Answer from the drawing. Dimensions are ordinates in mm from the lowest x, y and z of the part. A direction names the side the tool comes from. Give positions to 0.01 mm unless a question says otherwise; leave off trailing zeros. Write each loop counter-clockwise with the first axis right and the second up, starting at its lowest first coordinate (ties: lowest second). Pieces come first, ordered by that corner, then holes. Notation, with made-up numbers: M 75.5,9.25 L 131.5,9.25 A12 ccw 131.5,20.25 Z; hole C -14.5,5 d10. An arc over 180 degrees is marked long. Put each result on its own line as item: value.
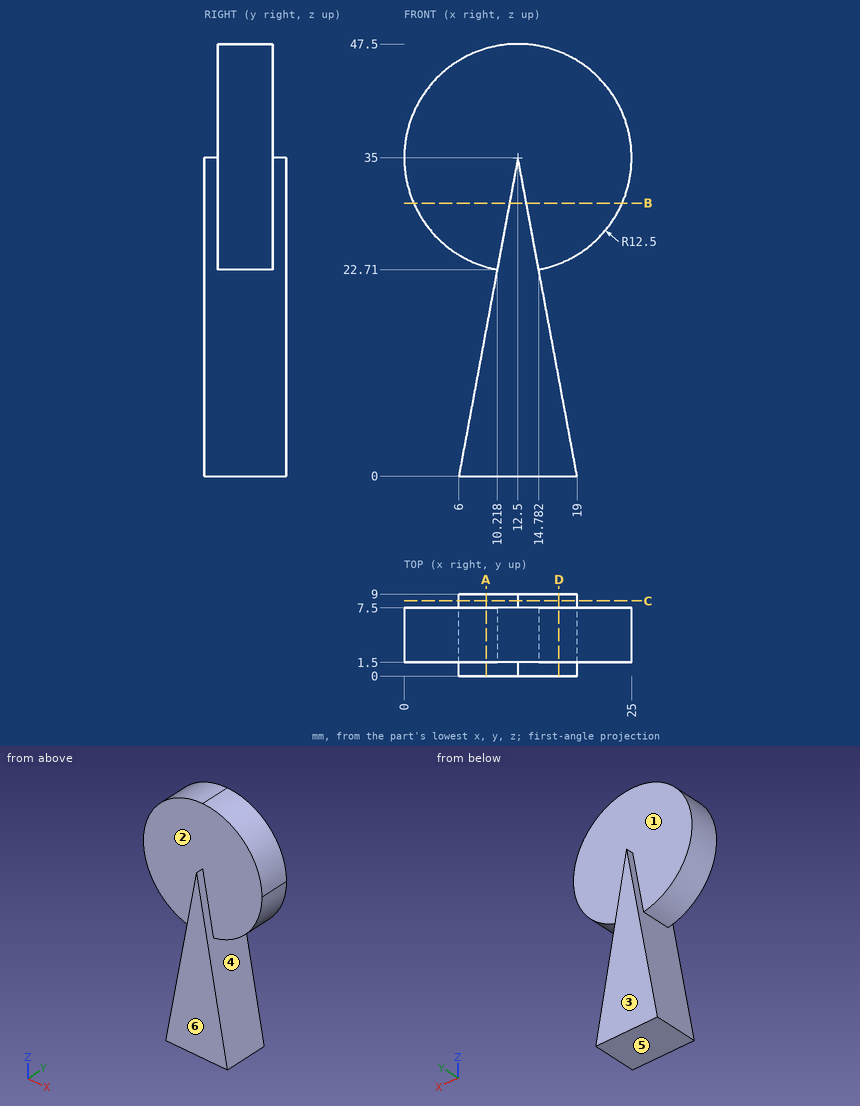
(1) Section C-C on y = 8.25 is taken. Determine the outline of the cut face in (x, z).
Result:
outline: M 6,0 L 19,0 L 12.5,35 Z
(2) Straight lines are drawn through the part: line 1 along Y through (x, z) = (6, 25.5); line 2 along Z through (x, y) = (12, 6.5); line 3 along Z through (x, y) = (22.5, 3.25). For each, find the intervals that lie inside material, in ascending order. Write a range as from..to.
Result:
line 1: y = 1.5..7.5
line 2: z = 0..47.49
line 3: z = 27.5..42.5
(3) Section B-B on z = 30 is taken. Determine the outline of the cut face in (x, y), and give its area (3 significant figures).
Result:
outline: M 1.04,1.5 L 11.57,1.5 L 11.57,0 L 13.43,0 L 13.43,1.5 L 23.96,1.5 L 23.96,7.5 L 13.43,7.5 L 13.43,9 L 11.57,9 L 11.57,7.5 L 1.04,7.5 Z
area: 143 mm²
(4) Which of the six approach directions +Z, -Z, +X, -X, +Y, -Y give full straight-line access (tool end or side, diameter ignored) to the marked faces 1, 2 and 3?
Result:
face 1: +Z, +Y
face 2: +Z, -Y
face 3: +Z, -Z, +X, -X, +Y
(5) Section D-D on x = 17 is taken. Determine the outline of the cut face in (y, z).
Result:
outline: M 0,0 L 9,0 L 9,10.77 L 0,10.77 Z; M 1.5,23.34 L 7.5,23.34 L 7.5,46.66 L 1.5,46.66 Z
(6) For a pull along Z with two mould halves and no side action, classify the marked faces 4, 5 and 6 as +Z half, -Z half, draft (parallel to the pull), parting line (faces both ways), or undercut.
Result:
face 4: undercut
face 5: -Z half
face 6: draft
(7) Section A-A on x = 9 is taken. Determine the outline of the cut face in (y, z).
Result:
outline: M 0,0 L 9,0 L 9,16.15 L 0,16.15 Z; M 1.5,23 L 7.5,23 L 7.5,47 L 1.5,47 Z
(8) Given pin 1 Ø4 at (x, z) = (4, 8) entering from -Y; pin 2 Ø1.5 at (y, z) = (3, 34) entering from +X; pin 3 Ø10 at (x, z) = (15, 42.5) entering from -Y; pin 4 Ø3 at (y, z) = (6, 9.5) entering from -X, each flat-ended and moving along its own axis, determine where each tip first touches the part or whether it passes through.
Result:
pin 1: passes through
pin 2: stops at x = 25
pin 3: stops at y = 1.5
pin 4: stops at x = 7.49
